Work out the finished part from the listing and answer in its coordinate system (mm). A direction names the side the tool comes from. Round coordinates to 2 decimals unless told otherwise and drop trailing zeros. Order: outer loops, then holes, each group sorted by start corner. A loop starts at its lowest first (then second) coordinate and runs counter-clockwise, first axis right, second up. Notation, with made-up numbers: (-31.75, 1.25) -> (25.25, 1.25) arc R28 cw to (25.25, 20.25) -> close; hole circle Ø4 at (35.25, 14.25). An arc over 180 degrees is marked (long way). Use one line per item in the form item = value.
Autodesk Inventor part; units mm, degrees
ref_plane "YZ Plane" through (0, 0, 0) normal (1, 0, 0) x (0, 1, 0)
ref_plane "XZ Plane" through (0, 0, 0) normal (0, 1, 0) x (-1, 0, 0)
ref_plane "XY Plane" through (0, 0, 0) normal (0, 0, 1) x (1, 0, 0)
sketch "スケッチ1" plane through (0, 0, 0) normal (0, 0, 1) x (1, 0, 0)
  line L0 (0, 0) -> (-65, 0)
  line L1 (-65, 0) -> (-65, -60)
  line L2 (-65, -60) -> (0, -60)
  line L3 (0, -60) -> (0, 0)
  dimension "d0" = 65
  dimension "d1" = 60
extrude "押し出し1" add sketch "スケッチ1" along normal blind 3
sketch "スケッチ2" plane through (0, 0, 3) normal (0, 0, 1) x (1, 0, 0)
  line L0 (-29, -25.6891) -> (-49.829, 0)
  line L1 (-2.171, 0) -> (-23, -25.6891)
  line L2 (-62, -31) -> (-65, -31)
  line L3 (-65, -31) -> (-65, -25)
  line L4 (-65, -25) -> (-62, -25)
  line L5 (-62, -25) -> (-62, -31)
  line L6 (-62, -17) -> (-65, -17)
  line L7 (-65, -17) -> (-65, -11)
  line L8 (-65, -11) -> (-62, -11)
  line L9 (-62, -11) -> (-62, -17)
  line L10 (-65, 4) -> (-62, 4)
  line L11 (-62, 4) -> (-62, 0)
  line L12 (-62, 0) -> (-65, 0)
  line L13 (-65, -4) -> (-65, 0)
  line L14 (-62, -4) -> (-65, -4)
  line L15 (-62, 0) -> (-62, -4)
  line L16 (-65, 0) -> (-65, 4)
  line L17 (-65, -40) -> (-62, -40)
  line L18 (0, 0) -> (0, -60)
  line L19 (0, -60) -> (-65, -60)
  line L20 (-65, -60) -> (-65, 0)
  line L21 (-65, 0) -> (0, 0)
  line L22 (-49.829, 0) -> (-62, -11)
  arc A0 (-29, -32.3891) -> (-23, -32.3891) centre (-26, -32.3891) ccw
  line L23 (-26, -32.3891) -> (-26, -29.3891) construction
  circle A1 centre (-26, -32.3891) radius 1.25
  line L24 (-23, -32.3891) -> (-23, -25.6891)
  line L25 (-29, -32.3891) -> (-29, -25.6891)
  circle A2 centre (-26, -18.3891) radius 1.25
  circle A3 centre (-26, -6.3891) radius 1.25
  line L26 (-29, -25.6891) -> (-62, -31)
  dimension "d4" = 6
  dimension "d5" = 2.5
  dimension "d6" = 3
  dimension "d7" = 2.5
  dimension "d8" = 2.5
  dimension "d9" = 14
  dimension "d10" = 26
extrude "押し出し2" cut sketch "スケッチ2" against normal blind 3 contours L26 L5 L4 L20 L6 L9 L22 L0 | L0 L21 L1 L24 A0 L25 keep common part
sketch "スケッチ3" plane through (0, 0, 3) normal (0, 0, 1) x (1, 0, 0)
  circle A0 centre (-26, -6.3891) radius 1.25
  circle A1 centre (-26, -18.3891) radius 1.25
  circle A2 centre (-26, -32.3891) radius 1.25
  line L0 (-62, -25) -> (-65, -25)
  line L1 (-65, -25) -> (-65, -17)
  line L2 (-65, -17) -> (-62, -17)
  line L3 (-62, -17) -> (-62, -11)
  line L4 (-62, -11) -> (-49.829, 0)
  line L5 (-49.829, 0) -> (-2.171, 0)
  line L6 (-2.171, 0) -> (-23, -25.6891)
  line L7 (-23, -25.6891) -> (-23, -32.3891)
  arc A3 (-29, -32.3891) -> (-23, -32.3891) centre (-26, -32.3891) ccw
  line L8 (-29, -32.3891) -> (-29, -25.6891)
  line L9 (-29, -25.6891) -> (-62, -31)
  line L10 (-62, -31) -> (-62, -25)
  arc A4 (-62, -28.9881) -> (-62, -27.7881) centre (-62.8, -28.3881) ccw
  arc A5 (-62, -14.6) -> (-62, -13.4) centre (-62.8, -14) ccw
  point P0 (0, 0)
  dimension "d13" = 2
  dimension "d14" = 2
  dimension "d15" = 3
  dimension "d16" = 3.3881
  dimension "d17" = 0.8
extrude "押し出し3" cut sketch "スケッチ3" against normal blind 3 contours A4 L10 | L3 A5
sketch "スケッチ4" plane through (0, 0, 3) normal (0, 0, 1) x (1, 0, 0)
  circle A0 centre (-26, -6.3891) radius 1.25
  circle A1 centre (-26, -18.3891) radius 1.25
  circle A2 centre (-26, -32.3891) radius 1.25
  line L0 (-29, -32.3891) -> (-29, -25.6891)
  line L1 (-29, -25.6891) -> (-62, -31)
  line L2 (-62, -31) -> (-62, -28.9881)
  arc A3 (-62, -28.9881) -> (-62, -27.7881) centre (-62.8, -28.3881) ccw
  line L3 (-62, -27.7881) -> (-62, -25)
  line L4 (-62, -25) -> (-65, -25)
  line L5 (-65, -25) -> (-65, -17)
  line L6 (-65, -17) -> (-62, -17)
  line L7 (-62, -17) -> (-62, -14.6)
  arc A4 (-62, -14.6) -> (-62, -13.4) centre (-62.8, -14) ccw
  line L8 (-62, -13.4) -> (-62, -11)
  line L9 (-62, -11) -> (-49.829, 0)
  line L10 (-49.829, 0) -> (-2.171, 0)
  line L11 (-2.171, 0) -> (-23, -25.6891)
  line L12 (-23, -25.6891) -> (-23, -32.3891)
  arc A5 (-29, -32.3891) -> (-23, -32.3891) centre (-26, -32.3891) ccw
  line L13 (-58, -25) -> (-61, -25)
  line L14 (-61, -25) -> (-61, -17)
  line L15 (-61, -17) -> (-58, -17)
  line L16 (-65, -17) -> (-65, -25)
  line L17 (-62, -25) -> (-65, -25)
  circle A6 centre (-58.8, -28.3881) radius 1
  circle A7 centre (-58.8, -14) radius 1
  arc A8 (-62, -14.6) -> (-62, -13.4) centre (-62.8, -14) ccw
  line L18 (-49.829, 0) -> (-58, -11)
  line L19 (-58, -31) -> (-29, -25.6891)
  line L20 (-29, -25.6891) -> (-49.829, 0)
  line L21 (-58, -31) -> (-58, -28.9881)
  line L22 (-58, -27.7881) -> (-58, -25)
  line L23 (-58, -17) -> (-58, -14.6)
  line L24 (-58, -13.4) -> (-58, -11)
  dimension "d26" = 3
  dimension "d27" = 6
  dimension "d28" = 6
  dimension "d29" = 4
sketch "スケッチ5" plane through (0, 0, 3) normal (0, 0, 1) x (1, 0, 0)
  circle A0 centre (-26, -6.3891) radius 1.25
  circle A1 centre (-26, -18.3891) radius 1.25
  circle A2 centre (-26, -32.3891) radius 1.25
  line L0 (-29, -32.3891) -> (-29, -25.6891)
  line L1 (-29, -25.6891) -> (-62, -31)
  line L2 (-62, -31) -> (-62, -28.9881)
  arc A3 (-62, -28.9881) -> (-62, -27.7881) centre (-62.8, -28.3881) ccw
  line L3 (-62, -27.7881) -> (-62, -25)
  line L4 (-62, -25) -> (-65, -25)
  line L5 (-65, -25) -> (-65, -17)
  line L6 (-65, -17) -> (-62, -17)
  line L7 (-62, -17) -> (-62, -14.6)
  arc A4 (-62, -14.6) -> (-62, -13.4) centre (-62.8, -14) ccw
  line L8 (-62, -13.4) -> (-62, -11)
  line L9 (-62, -11) -> (-49.829, 0)
  line L10 (-49.829, 0) -> (-2.171, 0)
  line L11 (-2.171, 0) -> (-23, -25.6891)
  line L12 (-23, -25.6891) -> (-23, -32.3891)
  arc A5 (-29, -32.3891) -> (-23, -32.3891) centre (-26, -32.3891) ccw
  circle A6 centre (-26, -6.3891) radius 1.25
  circle A7 centre (-26, -18.3891) radius 1.25
  circle A8 centre (-26, -32.3891) radius 1.25
  line L13 (-29, -32.3891) -> (-29, -25.6891)
  line L14 (-29, -25.6891) -> (-62, -31)
  line L15 (-62, -31) -> (-62, -28.9881)
  arc A9 (-62, -28.9881) -> (-62, -27.7881) centre (-62.8, -28.3881) ccw
  line L16 (-62, -27.7881) -> (-62, -25)
  line L17 (-62, -25) -> (-65, -25)
  line L18 (-65, -25) -> (-65, -17)
  line L19 (-65, -17) -> (-62, -17)
  line L20 (-62, -17) -> (-62, -14.6)
  arc A10 (-62, -14.6) -> (-62, -13.4) centre (-62.8, -14) ccw
  line L21 (-62, -13.4) -> (-62, -11)
  line L22 (-62, -11) -> (-49.829, 0)
  line L23 (-49.829, 0) -> (-2.171, 0)
  line L24 (-2.171, 0) -> (-23, -25.6891)
  line L25 (-23, -25.6891) -> (-23, -32.3891)
  arc A11 (-29, -32.3891) -> (-23, -32.3891) centre (-26, -32.3891) ccw
  circle A12 centre (-26, -6.3891) radius 1.25
  circle A13 centre (-26, -18.3891) radius 1.25
  circle A14 centre (-26, -32.3891) radius 1.25
  line L26 (-29, -32.3891) -> (-29, -25.6891)
  line L27 (-29, -25.6891) -> (-62, -31)
  line L28 (-62, -31) -> (-62, -28.9881)
  arc A15 (-62, -28.9881) -> (-62, -27.7881) centre (-62.8, -28.3881) ccw
  line L29 (-62, -27.7881) -> (-62, -25)
  line L30 (-62, -25) -> (-65, -25)
  line L31 (-65, -25) -> (-65, -17)
  line L32 (-65, -17) -> (-62, -17)
  line L33 (-62, -17) -> (-62, -14.6)
  arc A16 (-62, -14.6) -> (-62, -13.4) centre (-62.8, -14) ccw
  line L34 (-62, -13.4) -> (-62, -11)
  line L35 (-62, -11) -> (-49.829, 0)
  line L36 (-49.829, 0) -> (-2.171, 0)
  line L37 (-2.171, 0) -> (-23, -25.6891)
  line L38 (-23, -25.6891) -> (-23, -32.3891)
  arc A17 (-29, -32.3891) -> (-23, -32.3891) centre (-26, -32.3891) ccw
  arc A18 (-62, -14.6) -> (-62, -13.4) centre (-62.8, -14) ccw
  line L39 (-62, -17) -> (-62, -14.6)
  line L40 (-65, -17) -> (-62, -17)
  line L41 (-65, -17) -> (-65, -25)
  line L42 (-62, -25) -> (-65, -25)
  line L43 (-62, -27.7881) -> (-62, -25)
  arc A19 (-62, -28.9881) -> (-62, -27.7881) centre (-62.8, -28.3881) ccw
  line L44 (-62, -31) -> (-62, -28.9881)
  line L45 (-29, -25.6891) -> (-62, -31)
  line L46 (-29, -32.3891) -> (-29, -25.6891)
  arc A20 (-29, -32.3891) -> (-23, -32.3891) centre (-26, -32.3891) ccw
  line L47 (-23, -25.6891) -> (-23, -32.3891)
  line L48 (-2.171, 0) -> (-23, -25.6891)
  line L49 (-2.171, 0) -> (-49.829, 0)
  line L50 (-62, -11) -> (-49.829, 0)
  line L51 (-62, -13.4) -> (-62, -11)
  circle A21 centre (-26, -32.3891) radius 1.25
  circle A22 centre (-26, -18.3891) radius 1.25
  circle A23 centre (-26, -6.3891) radius 1.25
  line L52 (-29, -25.6891) -> (-49.829, 0)
  line L53 (-29, -25.6891) -> (-65.9346, -36.6422)
  line L54 (-65.9346, -36.6422) -> (-73.9425, -10.887)
  line L55 (-73.9425, -10.887) -> (-49.829, 0)
  point P0 (0, 0)
extrude "押し出し4" [suppressed]
extrude "押し出し5" [suppressed]
sketch "スケッチ6" plane through (0, 0, 0) normal (0, 0, -1) x (-1, 0, 0)
  circle A0 centre (26, -32.3891) radius 1.25
  circle A1 centre (26, -18.3891) radius 1.25
  circle A2 centre (26, -6.3891) radius 1.25
  arc A3 (62, -13.4) -> (62, -14.6) centre (62.8, -14) ccw
  line L0 (62, -11) -> (62, -13.4)
  line L1 (49.829, 0) -> (62, -11)
  line L2 (2.171, 0) -> (49.829, 0)
  line L3 (23, -25.6891) -> (2.171, 0)
  line L4 (23, -32.3891) -> (23, -25.6891)
  arc A4 (23, -32.3891) -> (29, -32.3891) centre (26, -32.3891) ccw
  line L5 (29, -25.6891) -> (29, -32.3891)
  line L6 (62, -31) -> (29, -25.6891)
  line L7 (62, -28.9881) -> (62, -31)
  arc A5 (62, -27.7881) -> (62, -28.9881) centre (62.8, -28.3881) ccw
  line L8 (62, -25) -> (62, -27.7881)
  line L9 (65, -25) -> (62, -25)
  line L10 (65, -17) -> (65, -25)
  line L11 (62, -17) -> (65, -17)
  line L12 (62, -14.6) -> (62, -17)
  point P0 (0, 0)
equation "\"d28\" = d27"
properties part number "handPlate"
Item 1: The part is cut by section B-B, the plane z = 1.9. Give the vertices of the cut face in (x, y).
Findings:
outline = (-65, -25) -> (-62, -25) -> (-62, -27.79) arc R1 cw to (-62, -28.99) -> (-62, -31) -> (-29, -25.69) -> (-29, -32.39) arc R3 ccw to (-23, -32.39) -> (-23, -25.69) -> (-2.17, 0) -> (-49.83, 0) -> (-62, -11) -> (-62, -13.4) arc R1 cw to (-62, -14.6) -> (-62, -17) -> (-65, -17) -> close; hole circle Ø2.5 at (-26, -32.39); hole circle Ø2.5 at (-26, -18.39); hole circle Ø2.5 at (-26, -6.39)
Item 2: Determine the mould class of faces 1 (the cylindrical face through (-25.328, -17.335, 1.521)), 2 (the flat face through (-34, -14, 0)), 3 (the flat face through (-64, -25, 2)) for opening direction Y: released by +Y, released by -Y, zero draft, split by the parting line, or undercut.
Findings:
face_1 = undercut
face_2 = zero draft
face_3 = released by -Y
Item 3: Consider line 1 along Y through (x, z) = (-26, 2.35); line 2 along X through (y, z) = (-18, 0.7); line 3 along Y through (x, z) = (-55, 0.25). Determine where each line is inside the solid, lowest interval first.
Findings:
line_1 = -35.39 to -33.64, -31.14 to -19.64, -17.14 to -7.64, -5.14 to 0
line_2 = -65 to -27.19, -24.81 to -16.77
line_3 = -29.87 to -4.67
Item 4: For faces 4 (the flat face through (-23, -29, 2)), 5 (the flat face through (-62, -12, 2)), 6 (the flat face through (-45.269, -28.307, 1.521)), 7 (the flat face through (-62, -26, 2)), determine the directions among +Z, -Z, +X, -X, +Y, -Y from which every point of the face is accessible in a straight line to the end or side of a thin tool.
Findings:
face_4 = +Z, -Z, +X, -Y
face_5 = +Z, -Z, -X, +Y
face_6 = +Z, -Z, -Y
face_7 = +Z, -Z, -X, -Y
Item 5: The part is cut by section C-C, the plane y = -22. Give the vertices of the cut face in (x, z).
Findings:
outline = (-65, 0) -> (-20.01, 0) -> (-20.01, 3) -> (-65, 3) -> close
Item 6: Flat-ended cylindrical pins translate along their axes: P1, Ø3, axis at x = -26, y = -6.39, coming from the -Z side; P2, Ø0.8, axis at y = -26, z = 1.5, coming from the -X side; P3, Ø1.5, axis at x = -64, z = 1.5, coming from the +Y side; P4, Ø1.5, axis at x = -32, z = 1.5, coming from the -Y side. Find the tip coordinate at first contact, or state that the pin passes through.
Findings:
P1 = 0
P2 = -62
P3 = -17
P4 = -26.29
Item 7: The part is cut by section D-D, the plane x = -34.5. Give the vertices of the cut face in (y, z), and give its area (3 significant figures).
Findings:
outline = (-26.57, 0) -> (0, 0) -> (0, 3) -> (-26.57, 3) -> close
area = 79.7 mm^2
Item 8: The part is cut by section A-A, the plane x = -26. Give the vertices of the cut face in (y, z).
Findings:
outline = (-35.39, 0) -> (-33.64, 0) -> (-33.64, 3) -> (-35.39, 3) -> close; (-31.14, 0) -> (-19.64, 0) -> (-19.64, 3) -> (-31.14, 3) -> close; (-17.14, 0) -> (-7.64, 0) -> (-7.64, 3) -> (-17.14, 3) -> close; (-5.14, 0) -> (0, 0) -> (0, 3) -> (-5.14, 3) -> close
